Read the model definition and answer for the solid it produces. Units are mm, in the model's axes. A direction names the side the tool comes from. Give positions to 0.01 mm unless a question says otherwise; leave off trailing zeros. Order: outer loops, then holes, each group sorted by start corner. A loop starts at its lowest first (then second) coordinate and runs counter-clockwise, first axis right, second up. Notation, with made-up numbers: (-23, 40.5) - (-14, 40.5) arc R14 ccw to (-14, 66.5) - close; hole circle Ø11 at (47.25, -9.5). An arc over 180 degrees is marked (long way). Use a Markdown table: item, result. Add a question column.
1. A cutting plane is placed at C-C on y = 0.55. State how many separate pieces and enclosed holes the cut face has, and give its area (3 significant figures).
2. Which of the six approach directions +Z, -Z, +X, -X, +Y, -Y give full straight-line access (tool end or side, diameter ignored) to faces 1 (the cylindrical face through (-12.63, 0.78, -53.34)), 2 (the flat face through (2, 2, 50.8))?
3. For a pull along X with two mould halves and no side action, classify faces 3 (the cylindrical face through (-16.723, 2.392, 6.901)), 4 (the cylindrical face through (24.805, 0.783, -40.563)), 5 (the flat face through (-11, 0, -55)), 6 (the flat face through (63.5, 2, -18)) as released by +X, released by -X, zero draft, split by the parting line, or undercut.
4. Consider L1, parallel to Z at x = -21, y = 2.7; L2, parallel to Z at x = 2, y = 1.35; L3, parallel to X at y = 2.75, z = 11.5. Determine where each line is inside the solid, lowest interval first.
5. A flat-ended cylindrical pin translates along its axis: P1, Ø3, axis at x = -12.32, z = -4.61, coming from the -Y side. Find the tip coordinate at first contact, or state that the pin passes through.
6. A cutting plane is placed at A-A on x = 8.5. Determine the outline of the cut face in (y, z) (1 decimal).
```python
from build123d import *

# Parameters (mm, degrees)
SKETCH1_W             = 101.6
SKETCH1_H             = 101.6
BOSS_EXTRUDE1_DEPTH   = 3.175
SKETCH3_W             = 50.8
SKETCH3_H             = 101.6
BOSS_EXTRUDE2_DEPTH   = 3.175
SKETCH6_W             = 152.4
SKETCH6_H             = 38.1
BOSS_EXTRUDE4_DEPTH   = 3.175
SKETCH9_W             = 6.35
SKETCH9_H             = 139.7
BOSS_EXTRUDE5_DEPTH   = 3.175
SKETCH7_OUTSIDE_W     = 203.048
SKETCH7_OUTSIDE_H     = 183.998
SKETCH7_OUTSIDE_W_2   = 120.65
SKETCH7_OUTSIDE_H_2   = 139.7
CUT_EXTRUDE3_DEPTH    = 4.175
F_4_40_TAPPED_HOLE2_D = 2.2606
SKETCH15_R            = 2.38125
CUT_EXTRUDE5_DEPTH    = 1.5875
FILLET1_R             = 3.429
F_2_56_TAPPED_HOLE_D  = 1.778
SKETCH19_R            = 2.4765
SKETCH19_R_2          = 0.889
BOSS_EXTRUDE6_DEPTH   = 1.5875
SKETCH21_R            = 5.55
CUT_EXTRUDE7_DEPTH    = 4.175
CUT_EXTRUDE8_DEPTH    = 2.5875
M2_CLEARANCE_HOLE1_D  = 2.2


with BuildPart() as part:
    # Sketch1 → Boss-Extrude1 (new body)
    with BuildSketch(Plane(origin=(0, 0, 0), x_dir=(1, 0, 0), z_dir=(0, 1, 0))):
        Rectangle(SKETCH1_W, SKETCH1_H)
    extrude(amount=BOSS_EXTRUDE1_DEPTH)

    # Sketch3 → Boss-Extrude2 (add)
    with BuildSketch(Plane(origin=(0, 3.175, 0), x_dir=(1, 0, 0), z_dir=(0, 1, 0))):
        with Locations((76.2, 0)):
            Rectangle(SKETCH3_W, SKETCH3_H)
    extrude(amount=-BOSS_EXTRUDE2_DEPTH)

    # Sketch6 → Boss-Extrude4 (add)
    with BuildSketch(Plane(origin=(0, 3.175, 0), x_dir=(1, 0, 0), z_dir=(0, 1, 0))):
        with Locations((25.4, 69.85)):
            Rectangle(SKETCH6_W, SKETCH6_H)
    extrude(amount=-BOSS_EXTRUDE4_DEPTH)

    # Sketch9 → Boss-Extrude5 (add)
    with BuildSketch(Plane(origin=(0, 3.175, 0), x_dir=(1, 0, 0), z_dir=(0, 1, 0))):
        with Locations((-53.975, 19.05)):
            Rectangle(SKETCH9_W, SKETCH9_H)
    extrude(amount=-BOSS_EXTRUDE5_DEPTH)

    # Sketch7 outside → Cut-Extrude3 (cut, through all)
    with BuildSketch(Plane(origin=(0, 3.175, 0), x_dir=(1, 0, 0), z_dir=(0, 1, 0))):
        with Locations((22.225, 19.05)):
            Rectangle(SKETCH7_OUTSIDE_W, SKETCH7_OUTSIDE_H)
        with Locations((3.175, 19.05)):
            Rectangle(SKETCH7_OUTSIDE_W_2, SKETCH7_OUTSIDE_H_2, mode=Mode.SUBTRACT)
    extrude(amount=-CUT_EXTRUDE3_DEPTH, mode=Mode.SUBTRACT)

    # #4-40 Tapped Hole2 (through all)
    with Locations(Plane(origin=(0, 3.175, 0), x_dir=(1, 0, 0), z_dir=(0, 1, 0))):
        with Locations((32.130819486, 46.000976371), (-2.794180514, 49.350976371), (-12.319180514, 55.700976371), (-21.844180514, 49.350976371), (22.605819486, 39.650976371), (41.655819486, 39.650976371), (-41.662637498, 9.355925684), (-41.662637498, -9.694074316), (-2.794180514, 73.025), (-12.319180514, 79.375), (-21.844180514, 73.025), (60.325, -47.625), (-53.975, -47.625), (60.325, 85.725), (-53.975, 85.725)):
            Hole(F_4_40_TAPPED_HOLE2_D / 2)

    # Sketch15 → Cut-Extrude5 (cut)
    with BuildSketch(Plane.XZ):
        with BuildLine():
            Line((-52.200121043, -87.3125), (58.550121043, -87.3125))
            ThreePointArc((58.550121043, -87.3125), (58.641201977, -84.041201977), (61.9125, -83.950121043))
            Line((61.9125, -83.950121043), (61.9125, 45.850121043))
            ThreePointArc((61.9125, 45.850121043), (58.641201977, 45.941201977), (58.550121043, 49.2125))
            Line((58.550121043, 49.2125), (-52.200121043, 49.2125))
            ThreePointArc((-52.200121043, 49.2125), (-52.291201977, 45.941201977), (-55.5625, 45.850121043))
            Line((-55.5625, 45.850121043), (-55.5625, -83.950121043))
            ThreePointArc((-55.5625, -83.950121043), (-52.291201977, -84.041201977), (-52.200121043, -87.3125))
        make_face()
        with Locations((32.130819486, -46.000976371)):
            Circle(SKETCH15_R, mode=Mode.SUBTRACT)
        with Locations((-2.794180514, -49.350976371)):
            Circle(SKETCH15_R, mode=Mode.SUBTRACT)
        with Locations((-12.319180514, -55.700976371)):
            Circle(SKETCH15_R, mode=Mode.SUBTRACT)
        with Locations((-21.844180514, -49.350976371)):
            Circle(SKETCH15_R, mode=Mode.SUBTRACT)
        with Locations((41.655819486, -39.650976371)):
            Circle(SKETCH15_R, mode=Mode.SUBTRACT)
        with Locations((22.605819486, -39.650976371)):
            Circle(SKETCH15_R, mode=Mode.SUBTRACT)
        with Locations((-41.662637498, 9.694074316)):
            Circle(SKETCH15_R, mode=Mode.SUBTRACT)
        with Locations((-41.662637498, -9.355925684)):
            Circle(SKETCH15_R, mode=Mode.SUBTRACT)
        with Locations((-2.794180514, -73.025)):
            Circle(SKETCH15_R, mode=Mode.SUBTRACT)
        with Locations((-12.319180514, -79.375)):
            Circle(SKETCH15_R, mode=Mode.SUBTRACT)
        with Locations((-21.844180514, -73.025)):
            Circle(SKETCH15_R, mode=Mode.SUBTRACT)
    extrude(amount=-CUT_EXTRUDE5_DEPTH, mode=Mode.SUBTRACT)

    # Fillet1
    fillet1_edges = [part.edges().sort_by_distance(p)[0] for p in [
        (-52.200121043, 0.79375, -87.3125),
        (-55.5625, 0.79375, -83.950121043),
        (-55.5625, 0.79375, 45.850121043),
        (-52.200121043, 0.79375, 49.2125),
        (58.550121043, 0.79375, 49.2125),
        (61.9125, 0.79375, 45.850121043),
        (61.9125, 0.79375, -83.950121043),
        (58.550121043, 0.79375, -87.3125),
    ]]
    fillet(fillet1_edges, radius=FILLET1_R)

    # #2-56 Tapped Hole (through all)
    with Locations(Plane(origin=(0, 3.175, 0), x_dir=(1, 0, 0), z_dir=(0, 1, 0))):
        with Locations((-0.819180486, 11.557600033), (-23.819180486, 11.557600033), (-0.819180486, 69.557600033), (-23.819180486, 69.557600033)):
            Hole(F_2_56_TAPPED_HOLE_D / 2)

    # Sketch19 → Boss-Extrude6 (add)
    with BuildSketch(Plane(origin=(0, 1.5875, 0), x_dir=(1, 0, 0), z_dir=(0, 1, 0))):
        with Locations((-23.819180486, 69.557600033)):
            Circle(SKETCH19_R)
        with Locations((-23.819180486, 69.557600033)):
            Circle(SKETCH19_R_2, mode=Mode.SUBTRACT)
        with Locations((-0.819180486, 69.557600033)):
            Circle(SKETCH19_R)
        with Locations((-0.819180486, 69.557600033)):
            Circle(SKETCH19_R_2, mode=Mode.SUBTRACT)
        with Locations((-23.819180486, 11.557600033)):
            Circle(SKETCH19_R)
        with Locations((-23.819180486, 11.557600033)):
            Circle(SKETCH19_R_2, mode=Mode.SUBTRACT)
        with Locations((-0.819180486, 11.557600033)):
            Circle(SKETCH19_R)
        with Locations((-0.819180486, 11.557600033)):
            Circle(SKETCH19_R_2, mode=Mode.SUBTRACT)
    extrude(amount=-BOSS_EXTRUDE6_DEPTH)

    # Sketch21 → Cut-Extrude7 (cut, through all)
    with BuildSketch(Plane(origin=(0, 3.175, 0), x_dir=(1, 0, 0), z_dir=(0, 1, 0))):
        with Locations((-12.319180514, -3.524023629)):
            Circle(SKETCH21_R)
    extrude(amount=-CUT_EXTRUDE7_DEPTH, mode=Mode.SUBTRACT)

    # Sketch22 → Cut-Extrude8 (cut, through all)
    with BuildSketch(Plane.XZ.offset(-1.5875)):
        with BuildLine():
            Line((-21.209180514, -85.471), (-3.429180514, -85.471))
            ThreePointArc((-3.429180514, -85.471), (-3.175180514, -85.725), (-3.429180514, -85.979))
            Line((-3.429180514, -85.979), (-21.209180514, -85.979))
            ThreePointArc((-21.209180514, -85.979), (-21.463180514, -85.725), (-21.209180514, -85.471))
        make_face()
    extrude(amount=-CUT_EXTRUDE8_DEPTH, mode=Mode.SUBTRACT)

    # M2 Clearance Hole1 (through all)
    with Locations(Plane(origin=(0, 3.175, 0), x_dir=(1, 0, 0), z_dir=(0, 1, 0))):
        with Locations((-20.450908498, -3.524023629), (-12.319180514, -11.655751612), (-4.187452531, -3.524023629), (-12.319180514, 4.607704355)):
            Hole(M2_CLEARANCE_HOLE1_D / 2)


solid = part.part
```
Output values:
| question | item | result |
|---|---|---|
| 1 | separate pieces | 14 |
| 1 | enclosed holes | 20 |
| 1 | area | 1,090 mm² |
| 2 | face 1 | -Y |
| 2 | face 2 | +Z, +X, -X, +Y, -Y |
| 3 | face 3 | undercut |
| 3 | face 4 | undercut |
| 3 | face 5 | zero draft |
| 3 | face 6 | released by +X |
| 4 | L1 | -88.9 to -85.98, -85.47 to -73.78, -72.27 to -50.1, -48.6 to 2.57, 4.48 to 50.8 |
| 4 | L2 | -88.9 to -87.31, 49.21 to 50.8 |
| 4 | L3 | -57.15 to -13.41, -11.23 to 63.5 |
| 5 | P1 | y = 1.59 |
| 6 | outline | (0, -88.9) - (3.2, -88.9) - (3.2, 50.8) - (0, 50.8) - (0, 49.2) - (1.6, 49.2) - (1.6, -87.3) - (0, -87.3) - close |
